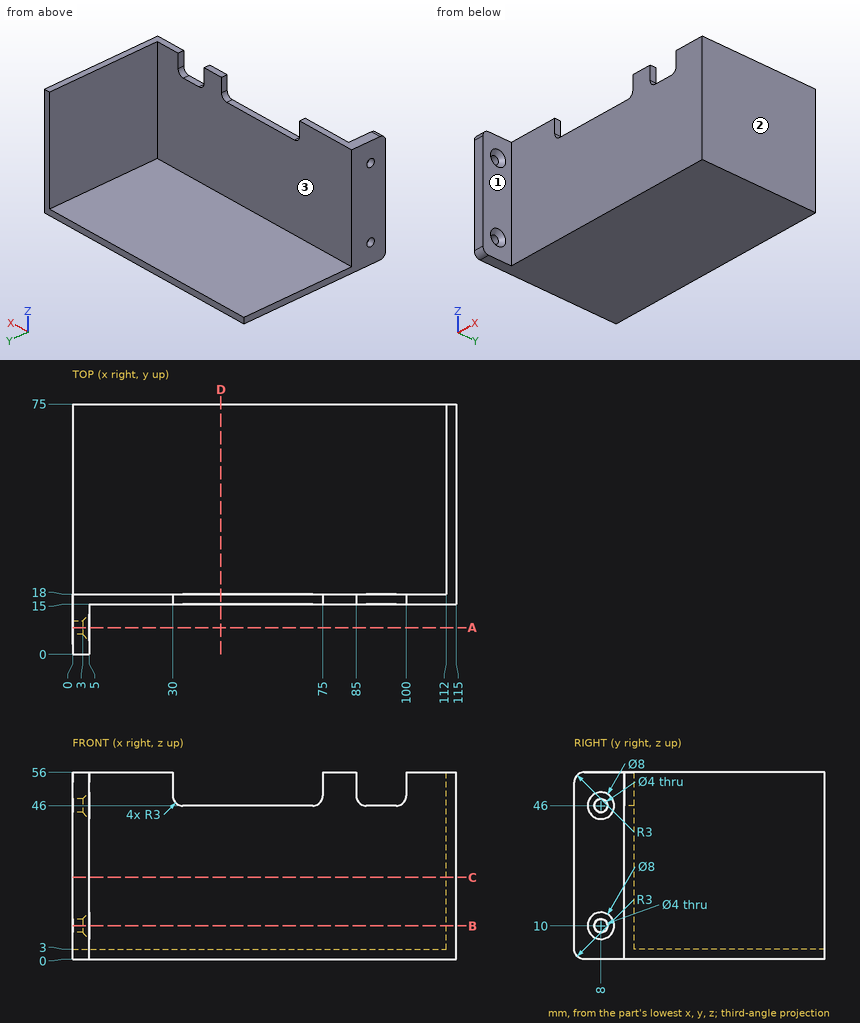
Geometry check sheet. Reference: drawing and pictorial views, mm from the part's lowest x, y, z. A direction names the side the tool comes from. Coordinates: 2 decimals unless noted, no trailing zeros. Write each loop counter-clockwise with the first axis right and the second up, starting at its lowest first coordinate (ties: lowest second). Pieces come first, ordered by that corner, then holes. Notation, with made-up numbers: (-9.75, -10.75) - (46.25, -10.75) arc R31 cw to (46.25, 20.25) - close; hole circle Ø10 at (52, 28.25). An arc over 180 degrees is marked (long way). One line per question, with ' | ' between items. Start each with the question number.
1. Access from +Z, -Z, +X, -X, +Y, -Y to the whole of each face (thin tool, end or side, straight path). Record for the marked faces 1, 2 and 3.
2. Material ranges on line 1 along Z through (x, y) = (0.9, 8); line 2 along Z through (x, y) = (53, 45); line 3 along Y through (x, z) = (100, 8), recorded low to high.
3. Section check B-B (z = 10). Enter the section's corners in (x, y).
4. Gauge pin test, flat ends, axial feed: P1, Ø2, axis at y = 26.5, z = 6, coming from the -X side; P2, Ø3, axis at y = 8, z = 46, coming from the +X side; P3, Ø1.5, axis at x = 48, y = 16, coming from the +Z side; P4, Ø12, axis at y = 5.5, z = 40, coming from the +X side. Record the tip position at first contact, or that the pin passes through.
5. Section check A-A (y = 8). Enter the section's corners in (x, z).
6. Section check C-C (z = 24.5). Enter the section's corners in (x, y), plus the area to 3 significant figures.
7. Section check D-D (x = 44.5). Enter the section's corners in (y, z), plus the area to 3 significant figures.
Computed values:
1) face 1: +Z, -Z, +X, -Y | face 2: +Z, -Z, +X, +Y, -Y | face 3: +Z, -X, +Y
2) line 1: 0 to 8, 12 to 44, 48 to 56 | line 2: 0 to 3 | line 3: 15 to 18
3) outline: (0, 0) - (5, 0) - (5, 4) - (3, 6) - (0, 6) - close; (0, 10) - (3, 10) - (5, 12) - (5, 15) - (115, 15) - (115, 75) - (112, 75) - (112, 18) - (0, 18) - close
4) P1: x = 112 | P2: through | P3: z = 46 | P4: x = 5
5) outline: (0, 0) - (5, 0) - (5, 6) - (3, 8) - (0, 8) - close; (0, 12) - (3, 12) - (5, 14) - (5, 42) - (3, 44) - (0, 44) - close; (0, 48) - (3, 48) - (5, 50) - (5, 56) - (0, 56) - close
6) outline: (0, 0) - (5, 0) - (5, 15) - (115, 15) - (115, 75) - (112, 75) - (112, 18) - (0, 18) - close | area: 591 mm²
7) outline: (15, 0) - (75, 0) - (75, 3) - (18, 3) - (18, 46) - (15, 46) - close | area: 309 mm²
